Can you work these out from the model? Positions are in its coordinate system, mm. Face numbers are marked on the shaded views. A direction names the side the tool comes from. Round coordinates to 2 decimals unless told otherwise and drop trailing zeros. Loops run counter-clockwise (first coordinate to the right, second up) from the corner with the lowest first, then second, coordinate; pieces in that order, holes last.
(1) Which directions (+Z, -Z, +X, -X, +Y, -Y) give clear straight access to the entire face, cutting with the end or side of a thin tool? Please do the marked faces 1 and 2.
(2) Will these pins go through, and if not, where does the flat tip stop? pin 1 Ø3 at (x, y) = (11.5, 41) entering from -Z; pin 2 Ø5 at (x, z) = (0.5, -38) entering from +Y.
(3) I want a section at A-A on x = 10. Write out the boundary of the cut face in (y, z), plus the area to 3 significant figures.
(4) I want a section at B-B on y = 19. Write out the boundary of the cut face in (x, z), plus the area to 3 significant figures.
(5) I want a section at C-C on z = -42. Write out the boundary of the cut face in (x, y).
(6) If I drill on line 1 along Z through (x, y) = (-3, 48); line 2 along Y through (x, z) = (-0.5, -14), over which ranges is the centre line in solid material (lowest first)?
from build123d import *

# Parameters (mm, degrees)
SKETCH1_W              = 35.052
SKETCH1_H              = 88.9
BASE_FLANGE1_DEPTH     = 1.21412
SKETCHED_START         = -17.526
SKETCHED_BEND1_DEPTH   = 35.052
SKETCHED_BEND1_2_DEPTH = 35.052


# Read off the part's stored shape, not the designer's step: Sketched Bend1
# Sheet-metal steps are written as plain solids
with BuildPart() as part:
    # Sketch1 → Base-Flange1 (new body)
    with BuildSketch(Plane(origin=(0, 0, 0), x_dir=(1, 0, 0), z_dir=(0, 1, 0))):
        Rectangle(SKETCH1_W, SKETCH1_H)
    extrude(amount=-BASE_FLANGE1_DEPTH)

    # Sketched Bend1 outline → Sketched Bend1 (cut)
    with BuildSketch(Plane.YZ.offset(SKETCHED_START)):
        with BuildLine():
            ThreePointArc((-1.21412, -7.405308096), (-0.882382531, -6.317096681), (0, -5.599005531))
            Line((0, -5.599005531), (0, 44.45))
            Line((0, 44.45), (-1.21412, 44.45))
            Line((-1.21412, 44.45), (-1.21412, -7.405308096))
        make_face()
    extrude(amount=SKETCHED_BEND1_DEPTH, mode=Mode.SUBTRACT)

    # Sketched Bend1 2 outline → Sketched Bend1 2 (add)
    with BuildSketch(Plane.YZ.offset(SKETCHED_START)):
        with BuildLine():
            Line((50.481291904, -6.668708096), (50.481291904, -5.454588096))
            Line((50.481291904, -5.454588096), (0.7366, -5.454588096))
            ThreePointArc((0.7366, -5.454588096), (0.361288145, -5.491032899), (0, -5.599005531))
            Line((0, -5.599005531), (0, -7.405308096))
            ThreePointArc((0, -7.405308096), (0.215745145, -6.884453241), (0.7366, -6.668708096))
            Line((0.7366, -6.668708096), (50.481291904, -6.668708096))
        make_face()
    extrude(amount=SKETCHED_BEND1_2_DEPTH)


solid = part.part
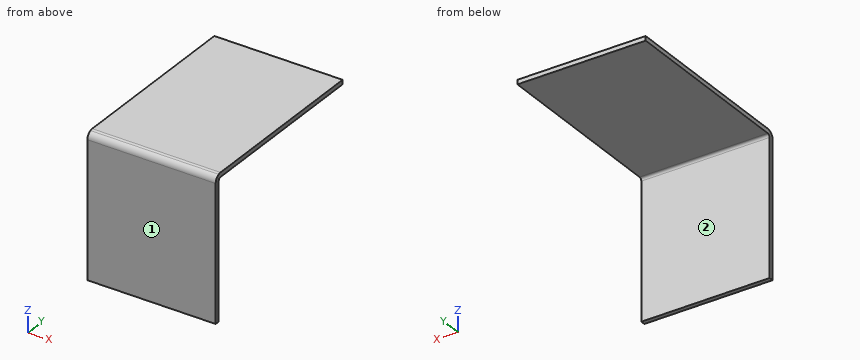
Filled sheet:
1. face 1: +Z, -Z, +X, -X, -Y
1. face 2: -Z, +X, -X, +Y
2. pin 1: stops at z = -6.67
2. pin 2: stops at y = 0
3. outline: (-1.21, -44.45) - (0, -44.45) - (0, -7.41) arc R0.74 cw to (0.74, -6.67) - (50.48, -6.67) - (50.48, -5.45) - (0.74, -5.45) arc R1.95 ccw to (-1.21, -7.41) - close
3. area: 108 mm2
4. outline: (-17.53, -6.67) - (17.53, -6.67) - (17.53, -5.45) - (-17.53, -5.45) - close
4. area: 42.6 mm2
5. outline: (-17.53, -1.21) - (17.53, -1.21) - (17.53, 0) - (-17.53, 0) - close
6. line 1: z = -6.67 to -5.45
6. line 2: y = -1.21 to 0
